Here's how the part is built. I have some questions about the finished solid (model axes, mm). Round coordinates to 2 decimals unless told otherwise and drop trailing zeros. Write each loop counter-clockwise with the first axis right and the second up, starting at its lowest first coordinate (ties: lowest second). Pieces come first, ordered by that corner, then holes. Notation, with made-up numbers: (44.5, 71.25) -> (100.5, 71.25) arc R20 ccw to (100.5, 105.25) -> close; hole circle Ø2 at (39.25, -30.5). An arc over 180 degrees is marked (long way). Put each result on its own line as item: value. Start each with the question number.
1) I want a section at A-A, the plane y = 10.5. List the corners of the cut face in (x, z) for me.
2) I want a section at B-B, the plane z = 0. Give the number of separate pieces and of enclosed holes in the cut face, then the cut area to 4 significant figures.
3) If I drill on line 1 along X through (y, z) = (6.25, 0); line 2 along X through (y, z) = (1.35, 0); line 3 along Z through (x, y) = (160, 1.65), over which ranges is the centre line in solid material (lowest first)? Write a range as [from, to].
4) Will these pins go through, and if not, where does the flat tip stop? P1, Ø8, axis at x = -40, z = 0, coming from the +Y side; P2, Ø5, axis at y = 1.5, z = 3, coming from the -X side; P3, Ø8, axis at y = 13, z = 6.5, coming from the -X side.
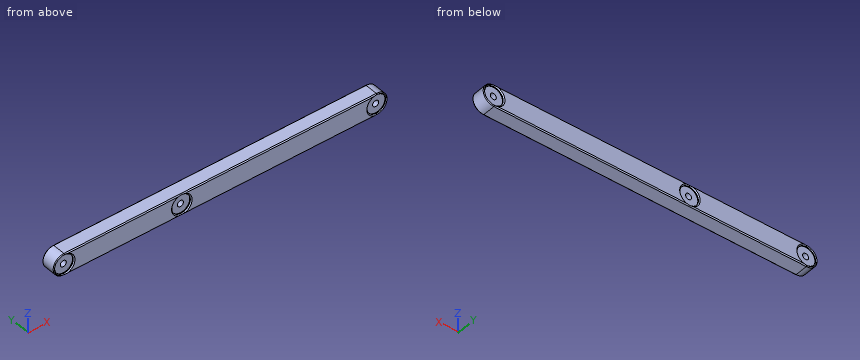
from build123d import *

# Parameters (mm, degrees)
SKETCH1_R           = 3.1
BOSS_EXTRUDE1_DEPTH = 15
SKETCH2_R           = 9.5
CUT_EXTRUDE1_DEPTH  = 1.8
CHAMFER2_SIZE       = 1


with BuildPart() as part:
    # Sketch1 → Boss-Extrude1 (new body)
    with BuildSketch(Plane(origin=(0, 0, 0), x_dir=(1, 0, 0), z_dir=(0, 1, 0))):
        with BuildLine():
            Line((-160, 11), (160, 11))
            ThreePointArc((160, 11), (171, 0), (160, -11))
            Line((160, -11), (-160, -11))
            ThreePointArc((-160, -11), (-171, 0), (-160, 11))
        make_face()
        with Locations(Location((-160, 0, 0), (0, 0, 270))):
            Circle(SKETCH1_R, mode=Mode.SUBTRACT)
        with Locations(Location((160, 0, 0), (0, 0, 270))):
            Circle(SKETCH1_R, mode=Mode.SUBTRACT)
        with Locations(Location((-40, 0, 0), (0, 0, 270))):
            Circle(SKETCH1_R, mode=Mode.SUBTRACT)
    extrude(amount=BOSS_EXTRUDE1_DEPTH)

    # Sketch2 → Cut-Extrude1 (cut)
    with BuildSketch(Plane(origin=(0, 15, 0), x_dir=(1, 0, 0), z_dir=(0, 1, 0))):
        with Locations(Location((160, 0, 0), (0, 0, 270))):
            Circle(SKETCH2_R)
        with Locations(Location((-40, 0, 0), (0, 0, 270))):
            Circle(SKETCH2_R)
        with Locations(Location((-160, 0, 0), (0, 0, 270))):
            Circle(SKETCH2_R)
    cut_extrude1 = extrude(amount=-CUT_EXTRUDE1_DEPTH, mode=Mode.SUBTRACT)

    # Chamfer2
    chamfer2_edges = [part.edges().sort_by_distance(p)[0] for p in [
        (171, 15, 0),
        (0, 15, -11),
        (-171, 15, 0),
        (0, 0, -11),
        (171, 0, 0),
        (0, 0, 11),
        (-171, 0, 0),
        (0, 15, 11),
    ]]
    chamfer(chamfer2_edges, length=CHAMFER2_SIZE)

    # Mirror1: Cut-Extrude1 across plane
    add(cut_extrude1.mirror(Plane.ZX.offset(7.5)), mode=Mode.SUBTRACT)

    # Chamfer1: read off the stored shape, not the designer's step
    # Chamfer1: loft between two sections, ruled curve by curve
    chamfer1_from = [
        Edge.make_three_point_arc((-160, 1, 9.5), (-169.5, 1, 0), (-160, 1, -9.5)),
        Edge.make_three_point_arc((-160, 1, -9.5), (-150.5, 1, 0), (-160, 1, 9.5)),
    ]
    chamfer1_to = [
        Edge.make_three_point_arc((-160, 0, 10.5), (-170.5, 0, 0), (-160, 0, -10.5)),
        Edge.make_three_point_arc((-160, 0, -10.5), (-149.5, 0, 0), (-160, 0, 10.5)),
    ]
    chamfer1 = Solid(Shell([*[Face.make_surface_from_curves(chamfer1_from[k], chamfer1_to[k]) for k in range(2)], Face(Wire(chamfer1_from)), Face(Wire(chamfer1_to))]))
    add(chamfer1, mode=Mode.SUBTRACT)

    # Chamfer1 2: loft between two sections, ruled curve by curve
    chamfer1_2_from = [
        Edge.make_three_point_arc((-37.103348559, 1, -9.047619048), (-30.952380952, 1, 2.896651441), (-42.896651441, 1, 9.047619048)),
        Edge.make_three_point_arc((-42.896651441, 1, 9.047619048), (-49.047619048, 1, -2.896651441), (-37.103348559, 1, -9.047619048)),
    ]
    chamfer1_2_to = [
        Edge.make_three_point_arc((-36.798437881, 0, -10), (-30, 0, 3.201562119), (-43.201562119, 0, 10)),
        Edge.make_three_point_arc((-43.201562119, 0, 10), (-50, 0, -3.201562119), (-36.798437881, 0, -10)),
    ]
    chamfer1_2 = Solid(Shell([*[Face.make_surface_from_curves(chamfer1_2_from[k], chamfer1_2_to[k]) for k in range(2)], Face(Wire(chamfer1_2_from)), Face(Wire(chamfer1_2_to))]))
    add(chamfer1_2, mode=Mode.SUBTRACT)

    # Chamfer1 3: loft between two sections, ruled curve by curve
    chamfer1_3_from = [
        Edge.make_three_point_arc((160, 1, 9.5), (150.5, 1, 0), (160, 1, -9.5)),
        Edge.make_three_point_arc((160, 1, -9.5), (169.5, 1, 0), (160, 1, 9.5)),
    ]
    chamfer1_3_to = [
        Edge.make_three_point_arc((160, 0, 10.5), (149.5, 0, 0), (160, 0, -10.5)),
        Edge.make_three_point_arc((160, 0, -10.5), (170.5, 0, 0), (160, 0, 10.5)),
    ]
    chamfer1_3 = Solid(Shell([*[Face.make_surface_from_curves(chamfer1_3_from[k], chamfer1_3_to[k]) for k in range(2)], Face(Wire(chamfer1_3_from)), Face(Wire(chamfer1_3_to))]))
    add(chamfer1_3, mode=Mode.SUBTRACT)

    # Chamfer1 4: loft between two sections, ruled curve by curve
    chamfer1_4_from = [
        Edge.make_three_point_arc((160, 14, 9.5), (169.5, 14, 0), (160, 14, -9.5)),
        Edge.make_three_point_arc((160, 14, -9.5), (150.5, 14, 0), (160, 14, 9.5)),
    ]
    chamfer1_4_to = [
        Edge.make_three_point_arc((160, 15, 10.5), (170.5, 15, 0), (160, 15, -10.5)),
        Edge.make_three_point_arc((160, 15, -10.5), (149.5, 15, 0), (160, 15, 10.5)),
    ]
    chamfer1_4 = Solid(Shell([*[Face.make_surface_from_curves(chamfer1_4_from[k], chamfer1_4_to[k]) for k in range(2)], Face(Wire(chamfer1_4_from)), Face(Wire(chamfer1_4_to))]))
    add(chamfer1_4, mode=Mode.SUBTRACT)

    # Chamfer1 5: loft between two sections, ruled curve by curve
    chamfer1_5_from = [
        Edge.make_three_point_arc((-40, 14, 9.5), (-30.5, 14, 0), (-40, 14, -9.5)),
        Edge.make_three_point_arc((-40, 14, -9.5), (-49.5, 14, 0), (-40, 14, 9.5)),
    ]
    chamfer1_5_to = [
        Edge.make_three_point_arc((-40, 15, 10.5), (-29.5, 15, 0), (-40, 15, -10.5)),
        Edge.make_three_point_arc((-40, 15, -10.5), (-50.5, 15, 0), (-40, 15, 10.5)),
    ]
    chamfer1_5 = Solid(Shell([*[Face.make_surface_from_curves(chamfer1_5_from[k], chamfer1_5_to[k]) for k in range(2)], Face(Wire(chamfer1_5_from)), Face(Wire(chamfer1_5_to))]))
    add(chamfer1_5, mode=Mode.SUBTRACT)

    # Chamfer1 6: loft between two sections, ruled curve by curve
    chamfer1_6_from = [
        Edge.make_three_point_arc((-160, 14, 9.5), (-150.5, 14, 0), (-160, 14, -9.5)),
        Edge.make_three_point_arc((-160, 14, -9.5), (-169.5, 14, 0), (-160, 14, 9.5)),
    ]
    chamfer1_6_to = [
        Edge.make_three_point_arc((-160, 15, 10.5), (-149.5, 15, 0), (-160, 15, -10.5)),
        Edge.make_three_point_arc((-160, 15, -10.5), (-170.5, 15, 0), (-160, 15, 10.5)),
    ]
    chamfer1_6 = Solid(Shell([*[Face.make_surface_from_curves(chamfer1_6_from[k], chamfer1_6_to[k]) for k in range(2)], Face(Wire(chamfer1_6_from)), Face(Wire(chamfer1_6_to))]))
    add(chamfer1_6, mode=Mode.SUBTRACT)


solid = part.part
Findings:
1. outline: (-160, -11) -> (160, -11) arc R11 ccw to (160, 11) -> (-160, 11) arc R11 ccw to start; hole circle Ø6.2 at (-160, 0); hole circle Ø6.2 at (-40, 0); hole circle Ø6.2 at (160, 0)
2. separate pieces: 4
2. enclosed holes: 0
2. area: 4,705 mm2
3. line 1: x = [-171, -163.1], [-156.9, -43.1], [-36.9, 156.9], [163.1, 171]
3. line 2: x = [-171, -169.5], [-150.5, -49.5], [-30.5, 150.5], [169.5, 171]
3. line 3: z = [-11, -9.5], [9.5, 11]
4. P1: stops at y = 13.2
4. P2: stops at x = -170.99
4. P3: stops at x = -170.71
